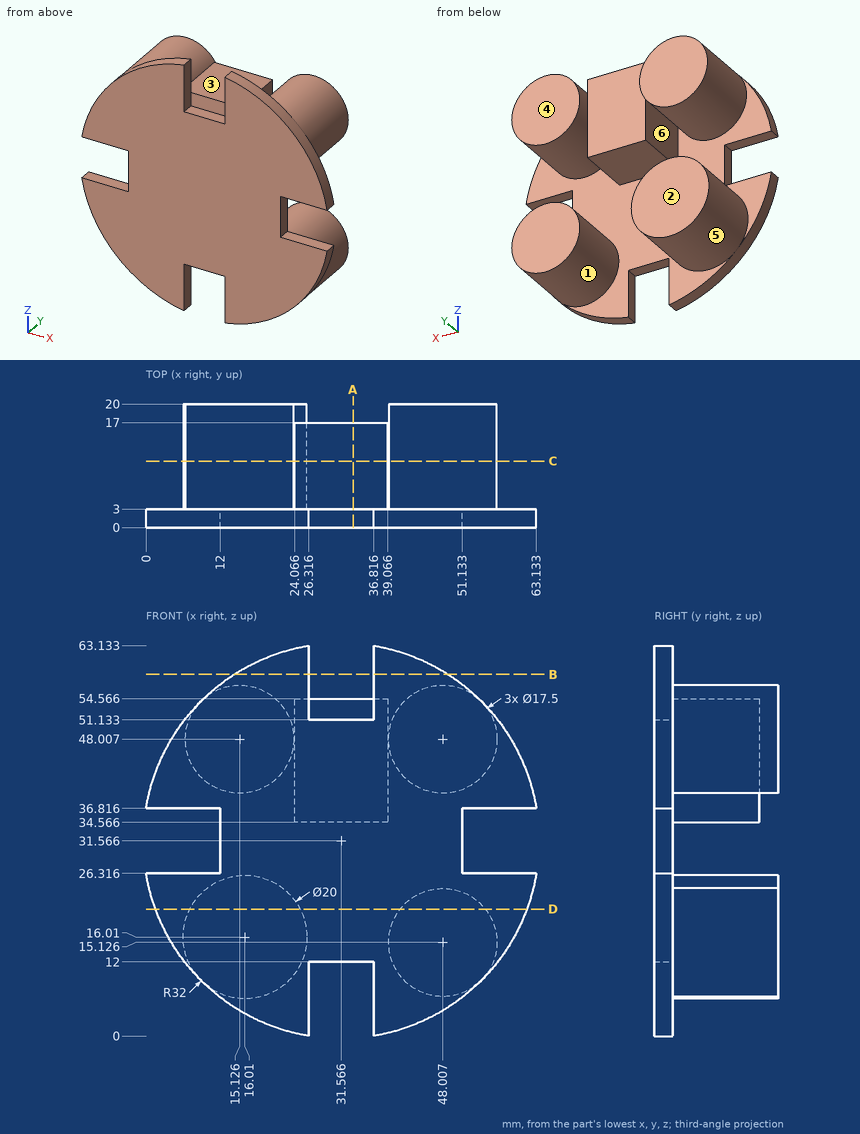
Geometry check sheet. Reference: drawing and pictorial views, mm from the part's lowest x, y, z. A direction names the side the tool comes from. Round coordinates to 2 decimals unless told otherwise and drop trailing zeros. Loops run counter-clockwise (first coordinate to the right, second up) from the corner with the lowest first, then second, coordinate; pieces in that order, holes last. Notation, with made-up numbers: (1.5, 9.25) -> (6.5, 9.25) arc R19 ccw to (6.5, 15.25) -> close; hole circle Ø4 at (26.5, -31). An arc over 180 degrees is marked (long way). Answer as a JSON object with one key per item and string values.
Q1. Scan lines: line 1 (X direction, y = 15, z = 45.5); line 2 (Y direction, x = 25.5, z = 3.5); line 3 (X direction, y = 14.5, z = 19). Record each from-to range of solid material in increasing order. Write a range as from..to.
Data:
{"line 1": "x = 6.74..23.51, 24.07..39.07, 39.62..56.39", "line 2": "y = 0..3", "line 3": "x = 6.47..25.55, 40.16..55.85"}
Q2. Section check B-B (z = 58.5). Record the boundary of the cut face in (x, y).
Data:
{"outline": "(14.29, 0) -> (26.32, 0) -> (26.32, 3) -> (14.29, 3) -> close; (36.82, 0) -> (48.85, 0) -> (48.85, 3) -> (36.82, 3) -> close"}
Q3. Section check D-D (z = 20.5). Record the boundary of the cut face in (x, y) (1 decimal).
Data:
{"outline": "(1.5, 0) -> (61.6, 0) -> (61.6, 3) -> (54.9, 3) -> (54.9, 20) -> (41.1, 20) -> (41.1, 3) -> (24.9, 3) -> (24.9, 20) -> (7.1, 20) -> (7.1, 3) -> (1.5, 3) -> close"}
Q4. Section check A-A (x = 33.5). Record the boundary of the cut face in (y, z).
Data:
{"outline": "(0, 12) -> (3, 12) -> (3, 34.57) -> (17, 34.57) -> (17, 54.57) -> (3, 54.57) -> (3, 51.13) -> (0, 51.13) -> close"}
Q5. Go/stop test with flat-tipped pins: P1, Ø6, axis at y = 5, z = 30, coming from the +X side; P2, Ø3.5, axis at y = 1, z = 57, coming from the +X side (1 decimal); P3, Ø12, axis at y = 3.5, z = 55, coming from the +X side. Record where each tip stops, or that it passes through.
Data:
{"P1": "stops at x = 51.13", "P2": "stops at x = 53.1", "P3": "stops at x = 58.39"}
Q6. Section check C-C (y = 10.75). Record the boundary of the cut face in (x, z), then the cut area to 3 significant figures.
Data:
{"outline": "circle Ø20 at (16.01, 16.01); circle Ø17.5 at (15.13, 48.01); (24.07, 34.57) -> (39.07, 34.57) -> (39.07, 54.57) -> (24.07, 54.57) -> close; circle Ø17.5 at (48.01, 15.13); circle Ø17.5 at (48.01, 48.01)", "area": "1,340 mm2"}
Q7. Access from +Z, -Z, +X, -X, +Y, -Y to the whole of each face (thin tool, end or side, straight path). Record for the marked faces 4, 5 and 6.
Data:
{"face 4": "+Z, -Z, +X, -X, +Y", "face 5": "+Y", "face 6": "+Z, +Y"}
Q8. Draft check along Z on the marked faces 1, 2 and 3. Enter one of: pulls with the +Z half, pulls with the -Z half, needs draft (parallel to the pull), parting line crosses it, or undercut.
Data:
{"face 1": "undercut", "face 2": "needs draft", "face 3": "pulls with the +Z half"}
